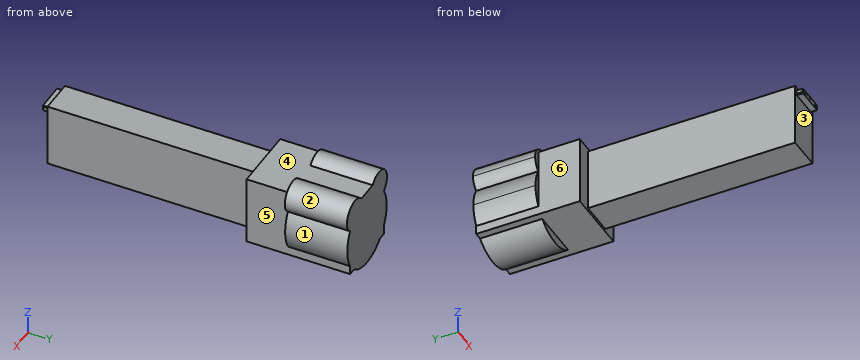
```python
from build123d import *

# Parameters (mm, degrees)
F0_W      = 41.4315387607
F0_H      = 78.3974006772
F1_DEPTH  = 254
F2_W      = 80.1340416074
F2_H      = 85.8401879668
F3_DEPTH  = 127
F4_W      = 33.4925614297
F4_H      = 6.4504221082
F5_DEPTH  = 7.62
F6_W      = 4.0796049871
F6_H      = 0.7493942976
F6_W_2    = 0.7494016
F7_DEPTH  = 0.1016
F8_R      = 1.27
F9_DEPTH  = 0.508
F10_W     = 0.762
F10_H     = 3.81
F11_DEPTH = 6.604
F13_DEPTH = 76.2


with BuildPart() as f1:
    # F0 (on Front) → F1 (new body)
    with BuildSketch(Plane.XZ):
        Rectangle(F0_W, F0_H)
    extrude(amount=F1_DEPTH)

    # F2 (on Front) → F3 (join)
    with BuildSketch(Plane.XZ):
        Rectangle(F2_W, F2_H)
    extrude(amount=-F3_DEPTH)

    # F4 (on face) → F5 (join)
    with BuildSketch(Plane.XZ.offset(254)):
        with Locations((0, 32.2520956397)):
            Rectangle(F4_W, F4_H)
    extrude(amount=F5_DEPTH)

    # F6 (on face) → F7 (cut)
    with BuildSketch(Plane.XZ.offset(261.62)):
        with Locations((0, 33.832609545)):
            Rectangle(F6_W, F6_H)
        with Locations((4.9545032935, 33.832609545)):
            Rectangle(F6_W_2, F6_H)
        with Locations((-4.9545032935, 33.832609545)):
            Rectangle(F6_W_2, F6_H)
    extrude(amount=-F7_DEPTH, mode=Mode.SUBTRACT)

    # F8 (on face) → F9 (join)
    with BuildSketch(Plane.XZ.offset(261.62)):
        with Locations((-11.6662807149, 31.5668845856)):
            Circle(F8_R)
        with Locations((11.6662807149, 31.5668845856)):
            Circle(F8_R)
    extrude(amount=F9_DEPTH)

    # F10 (on face) → F11 (join)
    with BuildSketch(Plane.XZ.offset(254)):
        with Locations((-17.1272807149, 32.3023066938)):
            Rectangle(F10_W, F10_H)
        with Locations((17.1272807149, 32.3023066938)):
            Rectangle(F10_W, F10_H)
    extrude(amount=F11_DEPTH)

    # F12 (on face) → F13 (join)
    with BuildSketch(Plane(origin=(0, 127, 0), x_dir=(-1, 0, 0), z_dir=(0, 1, 0))):
        with BuildLine():
            ThreePointArc((-40.2683013835, 16.40315221), (-20.2308740956, 14.3950889374), (-9.5870208037, 31.4900939834))
            ThreePointArc((-9.5870208037, 31.4900939834), (-9.8780164285, 34.807058688), (-10.7421131765, 38.0226877267))
            ThreePointArc((-10.7421131765, 38.0226877267), (-27.7013840338, 30.2122780312), (-40.2683013835, 16.40315221))
        make_face()
        with BuildLine():
            ThreePointArc((-10.7421131765, 38.0226877267), (-9.8780164285, 34.807058688), (-9.5870208037, 31.4900939834))
            ThreePointArc((-9.5870208037, 31.4900939834), (-20.2308740956, 14.3950889374), (-40.2683013835, 16.40315221))
            ThreePointArc((-40.2683013835, 16.40315221), (-12.4594875766, -52.8240828659), (46.8897423582, -7.62))
            ThreePointArc((46.8897423582, -7.62), (45.2040828659, 4.8394875766), (40.2683013835, 16.40315221))
            ThreePointArc((40.2683013835, 16.40315221), (17.3827178516, 16.1198901766), (10.7421131765, 38.0226877267))
            ThreePointArc((10.7421131765, 38.0226877267), (0, 39.2697423582), (-10.7421131765, 38.0226877267))
        make_face()
        with BuildLine():
            ThreePointArc((-40.2683013835, 16.40315221), (-27.7013840338, 30.2122780312), (-10.7421131765, 38.0226877267))
            ThreePointArc((-10.7421131765, 38.0226877267), (-39.8913237558, 46.8602977902), (-40.2683013835, 16.40315221))
        make_face()
        with BuildLine():
            ThreePointArc((40.2683013835, 16.40315221), (27.7013840338, 30.2122780312), (10.7421131765, 38.0226877267))
            ThreePointArc((10.7421131765, 38.0226877267), (17.3827178516, 16.1198901766), (40.2683013835, 16.40315221))
        make_face()
        with BuildLine():
            ThreePointArc((47.6870208037, 31.4900939834), (31.9539855082, 50.2490983586), (10.7421131765, 38.0226877267))
            ThreePointArc((10.7421131765, 38.0226877267), (27.7013840338, 30.2122780312), (40.2683013835, 16.40315221))
            ThreePointArc((40.2683013835, 16.40315221), (45.7320258497, 23.0839472754), (47.6870208037, 31.4900939834))
        make_face()
    extrude(amount=-F13_DEPTH)


solid = f1.part
```
Source: CAD feature listing. Evaluate the final solid. Frame: model axes, mm. Face numbers are marked on the shaded views. A direction names the side the tool comes from. Give positions to 0.01 mm unless a question says otherwise; leave off trailing zeros. Write each loop counter-clockwise with the first axis right and the second up, starting at its lowest first coordinate (ties: lowest second). Pieces come first, ordered by that corner, then holes. Notation, with made-up numbers: (-17, 89) - (-10, 89) arc R30 ccw to (-10, 128) - close; hole circle Ø11 at (48, 84). An arc over 180 degrees is marked (long way). One line per item, written item: value. Start each with the question number.
Q1. First-contact query: pin 1 Ø3 at (x, y) = (6, 26.5) entering from +Z; pin 2 Ø6 at (x, y) = (1.5, -195) entering from +Z; pin 3 Ø6 at (x, z) = (-0.5, -50.5) entering from -Y; pin 4 Ø12 at (x, y) = (27.5, -146.5) entering from +Z. Flat tips, straight axial feed; report the tip coordinate or a pass-through.
Q2. Section query C-C, the plane x = -26. Return the cut outline in (y, z), then the cut area to 3 significant figures.
Q3. Section query D-D, the plane z = 1. Return the cut outline in (x, y), then the cut area to 3 significant figures.
Q4. Draft query along X for the marked faces 1, 2 and 3. Return one class per face: +X half, -X half, draft (parallel to the pull), parting line (faces both ways), or undercut.
Q5. Set-up query: the marked faces 4, 5 and 6. Return all of +Z, -Z, +X, -X, +Y, -Y with unobstructed straight access to the full face (end or side cutting, diameter ignored); none if empty.
Q6. Material intervals for probe 1 along Y at (x, z) = (-5, -22); probe 2 along X at (y, z) = (33, 0); probe 3 along Y at (x, z) = (29.5, 17.5), sorted ascending. Write a range as from..to.
Q7. Section query B-B, the plane y = -87. Return the cut outline in (x, z).
Q8. Section query A-A, the plane z = -16.5. Return the cut outline in (x, y).
Answer:
1. pin 1: stops at z = 42.92
1. pin 2: stops at z = 39.2
1. pin 3: stops at y = 50.8
1. pin 4: passes through
2. outline: (0, -42.92) - (50.8, -42.92) - (50.8, -46.64) - (127, -46.64) - (127, 50.36) - (50.8, 50.36) - (50.8, 42.92) - (0, 42.92) - close
2. area: 11,800 mm2
3. outline: (-46.09, 50.8) - (-40.07, 50.8) - (-40.07, 0) - (-20.72, 0) - (-20.72, -254) - (20.72, -254) - (20.72, 0) - (40.07, 0) - (40.07, 50.8) - (46.09, 50.8) - (46.09, 127) - (-46.09, 127) - close
3. area: 21,600 mm2
4. face 1: +X half
4. face 2: undercut
4. face 3: draft
5. face 4: +Z, -Y
5. face 5: -Z, +X, -Y
5. face 6: -Z, -X, -Y
6. probe 1: y = -254..127
6. probe 2: x = -40.07..40.07
6. probe 3: y = 0..127
7. outline: (-20.72, -39.2) - (20.72, -39.2) - (20.72, 39.2) - (-20.72, 39.2) - close
8. outline: (-46.04, 50.8) - (-40.07, 50.8) - (-40.07, 0) - (-20.72, 0) - (-20.72, -254) - (20.72, -254) - (20.72, 0) - (40.07, 0) - (40.07, 50.8) - (46.04, 50.8) - (46.04, 127) - (-46.04, 127) - close
